```python
from build123d import *

# Parameters (mm, degrees)
PAD_DEPTH            = 16
SKETCH014_R          = 3.25
POCKET007_DEPTH      = 40
SKETCH015_R          = 4.5
POCKET008_DEPTH      = 45.501
POCKET008_DEPTH_BACK = -5.001
POCKET009_DEPTH      = 25.251


with BuildPart() as part:
    # Sketch → Pad (new body, symmetric)
    with BuildSketch(Plane.YZ):
        with BuildLine():
            Line((3, 0), (37.5, 0))
            ThreePointArc((40.5, -3), (39.62132, -0.87868), (37.5, 0))
            Line((40.5, -3), (40.5, -35))
            Line((40.5, -35), (42.5, -35))
            ThreePointArc((42.5, -35), (44.62132, -34.12132), (45.5, -32))
            Line((45.5, -32), (45.5, 22))
            ThreePointArc((45.5, 22), (43.156854, 27.656854), (37.5, 30))
            Line((3, 30), (37.5, 30))
            ThreePointArc((3, 30), (-2.656854, 27.656854), (-5, 22))
            Line((-5, -32), (-5, 22))
            ThreePointArc((-5, -32), (-4.12132, -34.12132), (-2, -35))
            Line((0, -35), (-2, -35))
            Line((0, -3), (0, -35))
            ThreePointArc((3, 0), (0.87868, -0.87868), (0, -3))
        make_face()
        with BuildLine():
            ThreePointArc((3, 25), (0.87868, 24.12132), (0, 22))
            Line((0, 8), (0, 22))
            ThreePointArc((0, 8), (0.87868, 5.87868), (3, 5))
            Line((37.5, 5), (3, 5))
            ThreePointArc((37.5, 5), (39.62132, 5.87868), (40.5, 8))
            Line((40.5, 22), (40.5, 8))
            ThreePointArc((40.5, 22), (39.62132, 24.12132), (37.5, 25))
            Line((3, 25), (37.5, 25))
        make_face(mode=Mode.SUBTRACT)
    extrude(amount=PAD_DEPTH, both=True)

    # Sketch014 → Pocket007 (cut)
    with BuildSketch(Plane.XY.offset(50)):
        with Locations((0, 20)):
            Circle(SKETCH014_R)
    extrude(amount=-POCKET007_DEPTH, mode=Mode.SUBTRACT)

    # Sketch015 → Pocket008 (cut, two sides)
    with BuildSketch(Plane.XZ) as pocket008_sk:
        with Locations((0, -20.25)):
            Circle(SKETCH015_R)
    extrude(amount=-POCKET008_DEPTH, mode=Mode.SUBTRACT)
    extrude(pocket008_sk.sketch, amount=-POCKET008_DEPTH_BACK, mode=Mode.SUBTRACT)

    # Sketch016 → Pocket009 (cut, through all)
    with BuildSketch(Plane.XZ.offset(-20.25)):
        Polygon((-56, 5), (-16, 5), (-5, 7.947441), (-5, 12.052559), (-16, 15), (-56, 15), align=None)
        Polygon((5, 12.052559), (5, 7.947441), (16, 5), (56, 5), (56, 15), (16, 15), align=None)
    extrude(amount=-POCKET009_DEPTH, mode=Mode.SUBTRACT)


solid = part.part
```
Geometry check sheet. Reference: the model listing, model coordinates, mm. A direction names the side the tool comes from. Round coordinates to 2 decimals unless told otherwise and drop trailing zeros. Loops run counter-clockwise (first coordinate to the right, second up) from the corner with the lowest first, then second, coordinate; pieces in that order, holes last. Notation, with made-up numbers: M 67.25,-26.75 L 76.25,-26.75 A17 ccw 76.25,-21.75 Z; hole C 30.25,43 d5. An arc over 180 degrees is marked long. Return JSON: item names as keys, results as strings. Group by question number.
(1) Set-up check for faces 5 (the face through (10.4, 42.3, 6.5)), 6 (the face through (4, 20, 25)), 7 (the face through (0, 20, 0)): record each of +Z, -Z, +X, -X, +Y, -Y from which the full face is reachable in a straight line by a thin tool's end or side.
(2) Section check C-C, the plane z = -20.25. Enter the section's corners in (x, y).
(3) Scan lines: line 1 along Z through (x, y) = (11, 16); line 2 along Y through (x, z) = (-11, 15); line 3 along X through (y, z) = (-2, -20). Record each from-to range of solid material in increasing order. Write a range as [from, to].
(4) Mould release check, pull along Y, two halves, no side actions. Record for faces 1 (the face through (-5, 43, 10)), 2 (the face through (0, 45.5, -5)), 3 (the face through (0, 0, -15)), 4 (the face through (0, -5, -5)): pulls with the +Y half, pulls with the -Y half, needs draft (parallel to the pull), parting line crosses it, or undercut.
(5) Section check B-B, the plane x = 0. Give the number of separate pieces and of enclosed holes in the cut face, and give its area (3 significant figures).
(6) Section check A-A, the plane y = 27.5. Enter the section's corners in (x, z).
(7) Go/stop test with flat-tipped pins: pin 1 (16 mm diameter, centred on x = -5, y = 21.5, fed in from -Z); pin 2 (3 mm diameter, centred on x = -12.5, z = 10.5, fed in from +Y); pin 3 (1.2 mm diameter, centred on y = 42, z = 9.5, fed in from -X). Record where each tip stops, or that it passes through.
(8) Section check D-D, the plane z = -29. Enter the section's corners in (x, y).
Data:
{
 "1": {"face 5": "+X, +Y", "face 6": "+X, -X", "face 7": "-Z, +X, -X"},
 "2": {"outline": "M -16,-5 L -4.5,-5 L -4.5,0 L -16,0 Z; M -16,40.5 L -4.5,40.5 L -4.5,45.5 L -16,45.5 Z; M 4.5,-5 L 16,-5 L 16,0 L 4.5,0 Z; M 4.5,40.5 L 16,40.5 L 16,45.5 L 4.5,45.5 Z"},
 "3": {"line 1": "[0, 5], [25, 30]", "line 2": "[-5, 0], [40.5, 45.5]", "line 3": "[-16, -4.49], [4.49, 16]"},
 "4": {"face 1": "needs draft", "face 2": "pulls with the +Y half", "face 3": "undercut", "face 4": "pulls with the -Y half"},
 "5": {"separate pieces": "3", "enclosed holes": "0", "area": "913 mm²"},
 "6": {"outline": "M -16,0 L 16,0 L 16,5 L -16,5 Z; M -16,25 L 16,25 L 16,30 L -16,30 Z"},
 "7": {"pin 1": "z = 0", "pin 2": "y = 0", "pin 3": "x = -5"},
 "8": {"outline": "M -16,-5 L 16,-5 L 16,0 L -16,0 Z; M -16,40.5 L 16,40.5 L 16,45.5 L -16,45.5 Z"}
}
